Geometry check sheet. Reference: drawing and pictorial views, mm from the part's lowest x, y, z. Coordinates: 2 decimals unless noted, no trailing zeros. Order: outer loops, then holes, each group sorted by start corner. A loop starts at its lowest first (then second) coordinate and runs counter-clockwise, first axis right, second up. Notation, with made-up numbers: (3, 65) -> (30, 65) arc R18 cw to (30, 94) -> close; hole circle Ø10 at (13.25, 16.5). An arc over 180 degrees is marked (long way). Use CSV: the item, a comma, the result in double quotes. Start each with the question number.
1) Sectioned sample at C-C on z = 1.25. Record the boundary of the cut face in (x, y) (3 decimals), then the cut area to 3 significant figures.
2) Sectioned sample at B-B on x = 64. Record the boundary of the cut face in (y, z) (3 decimals), then the cut area to 4 significant figures.
3) Sectioned sample at A-A on y = 44.5. Record the boundary of the cut face in (x, z) (3 decimals).
4) Scan lines: line 1 along X through (y, z) = (39.5, 0.95); line 2 along X through (y, z) = (3, 2.45); line 3 along Y through (x, z) = (66.5, 1.5). Record each from-to range of solid material in increasing order.
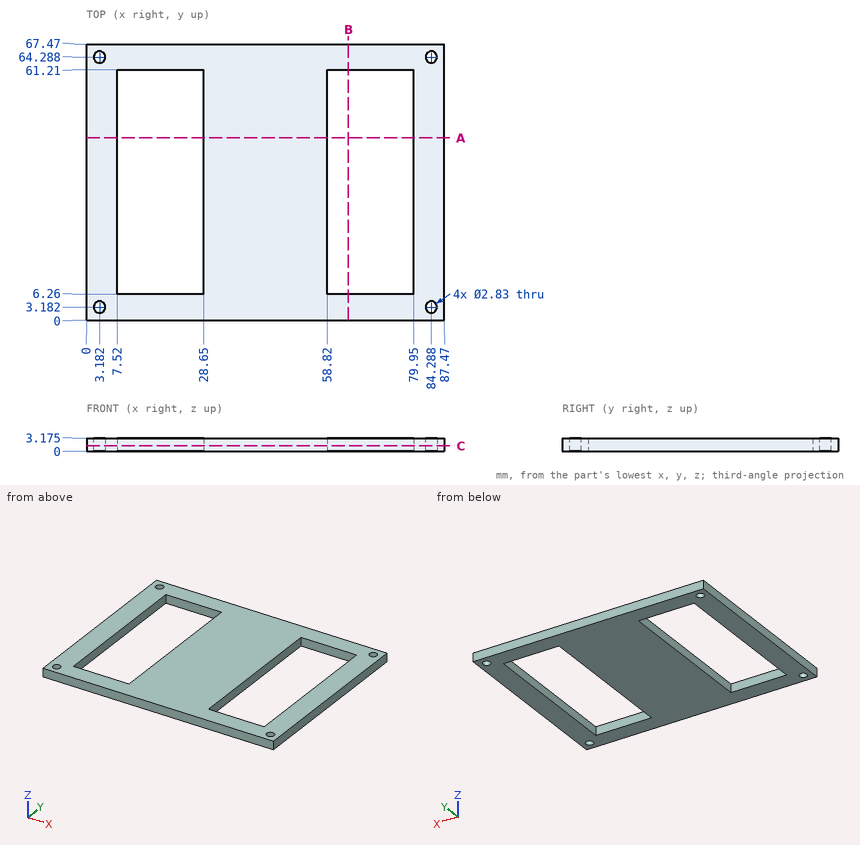
Answers follow:
1,outline,"(0, 0) -> (87.47, 0) -> (87.47, 67.47) -> (0, 67.47) -> close; hole circle Ø2.83 at (3.182, 3.182); hole circle Ø2.83 at (3.182, 64.288); hole (7.52, 6.26) -> (28.65, 6.26) -> (28.65, 61.21) -> (7.52, 61.21) -> close; hole (58.82, 6.26) -> (79.95, 6.26) -> (79.95, 61.21) -> (58.82, 61.21) -> close; hole circle Ø2.83 at (84.288, 3.182); hole circle Ø2.83 at (84.288, 64.288)"
1,area,"3,550 mm²"
2,outline,"(0, 0) -> (6.26, 0) -> (6.26, 3.175) -> (0, 3.175) -> close; (61.21, 0) -> (67.47, 0) -> (67.47, 3.175) -> (61.21, 3.175) -> close"
2,area,"39.75 mm²"
3,outline,"(0, 0) -> (7.52, 0) -> (7.52, 3.175) -> (0, 3.175) -> close; (28.65, 0) -> (58.82, 0) -> (58.82, 3.175) -> (28.65, 3.175) -> close; (79.95, 0) -> (87.47, 0) -> (87.47, 3.175) -> (79.95, 3.175) -> close"
4,line 1,"x = 0 to 7.52, 28.65 to 58.82, 79.95 to 87.47"
4,line 2,"x = 0 to 1.78, 4.59 to 82.88, 85.69 to 87.47"
4,line 3,"y = 0 to 6.26, 61.21 to 67.47"
